```python
from build123d import *

# Parameters (mm, degrees)
SKETCH_1_W      = 90
SKETCH_1_H      = 36
SKETCH_1_R      = 6
EXTRUDE_1_DEPTH = 16
EXTRUDE_2_DEPTH = 20
FILLET_1_R      = 1
FILLET_2_R      = 1


with BuildPart() as part:
    # Эскиз1 → Бобышка-Вытянуть1 (new body)
    with BuildSketch(Plane(origin=(0, 0, 0), x_dir=(1, 0, 0), z_dir=(0, 1, 0))):
        Rectangle(SKETCH_1_W, SKETCH_1_H)
        with Locations(Location((-6, 0, 0), (0, 0, 270))):
            Circle(SKETCH_1_R, mode=Mode.SUBTRACT)
    extrude(amount=EXTRUDE_1_DEPTH)

    # Эскиз3 → Бобышка-Вытянуть2 (add)
    with BuildSketch(Plane(origin=(0, 18, 0), x_dir=(1, 0, 0), z_dir=(0, 1, 0))):
        with BuildLine():
            Line((-45, 20.5), (-45, -20.5))
            Line((-45, -20.5), (-48, -20.5))
            Line((-48, -20.5), (-48, -9.285164832))
            ThreePointArc((-48, -9.285164832), (-48.252071986, -6.546804135), (-48.999815907, -3.900478642))
            Line((-48.999815907, -3.900478642), (-52.000184093, 3.900478642))
            ThreePointArc((-52.000184093, 3.900478642), (-52.747928014, 6.546804135), (-53, 9.285164832))
            Line((-53, 9.285164832), (-53, 19))
            ThreePointArc((-53, 19), (-52.560660172, 20.060660172), (-51.5, 20.5))
            Line((-51.5, 20.5), (-45, 20.5))
        make_face()
    extrude(amount=-EXTRUDE_2_DEPTH)

    # Скругление1
    fillet_1_edges = [part.edges().sort_by_distance(p)[0] for p in [
        (-48.25, 18, -20.5),
        (-52.560660172, 18, -20.060660172),
        (-53, 18, -14.142582416),
        (-52.747928014, 18, -6.546804135),
        (-50.5, 18, 0),
        (-48.252071986, 18, 6.546804135),
        (-48, 18, 14.892582416),
        (-46.5, 18, 20.5),
    ]]
    fillet(fillet_1_edges, radius=FILLET_1_R)

    # Скругление2
    fillet_2_edges = [part.edges().sort_by_distance(p)[0] for p in [
        (-45, -2, 0),
        (-48.25, -2, -20.5),
        (-46.5, -2, 20.5),
        (-48, -2, 14.892582416),
        (-48.252071986, -2, 6.546804135),
        (-50.5, -2, 0),
        (-52.747928014, -2, -6.546804135),
        (-53, -2, -14.142582416),
        (-52.560660172, -2, -20.060660172),
    ]]
    fillet(fillet_2_edges, radius=FILLET_2_R)


solid = part.part
```
Source: CAD feature listing. Evaluate the final solid. Frame: model axes, mm. A direction names the side the tool comes from. Coordinates: 2 decimals unless noted, no trailing zeros. Write each loop counter-clockwise with the first axis right and the second up, starting at its lowest first coordinate (ties: lowest second). Pieces come first, ordered by that corner, then holes. Notation, with made-up numbers: (63, 44.5) - (77, 44.5) arc R34 ccw to (77, 75.5) - close; hole circle Ø5 at (33.25, 44). An arc over 180 degrees is marked (long way). Answer as a JSON object with one key per item and string values.
Q1. Draft query along Z for faces 5 (the cylindrical face through (-11.323, 7.888, 2.769)), 6 (the cylindrical face through (-50.255, -1.699, -0.157)), 7 (the flat face through (-48, -2, -5)). Return one class per face: released by +Z, released by -Z, zero draft, split by the parting line, or undercut.
Ans:
{"face 5": "undercut", "face 6": "released by +Z", "face 7": "zero draft"}
Q2. Section query B-B, the plane y = 14. Output: boundary loops of the cut face in (x, z), plus the area to 3 significant figures.
Ans:
{"outline": "(-53, -19) arc R1.5 ccw to (-51.5, -20.5) - (-45, -20.5) - (-45, -18) - (45, -18) - (45, 18) - (-45, 18) - (-45, 20.5) - (-48, 20.5) - (-48, 9.29) arc R15 cw to (-49, 3.9) - (-52, -3.9) arc R15 ccw to (-53, -9.29) - close; hole circle Ø12 at (-6, 0)", "area": "3,350 mm2"}
Q3. Material intervals for line 1 (Z direction, x = 15, y = 12); line 2 (Y direction, x = -1, z = -3.5); line 3 (X direction, y = 5.25, z = 0), sorted ascending. Write a range as [from, to].
Ans:
{"line 1": "z = [-18, 18]", "line 2": "y = [0, 16]", "line 3": "x = [-50.5, -12], [0, 45]"}
Q4. First-contact query: pin 1 Ø1 at (x, y) = (-17.5, 12.5) entering from +Z; pin 2 Ø2 at (y, z) = (7, 7.5) entering from -X; pin 3 Ø1.5 at (x, y) = (-39.5, 10) entering from -Z. Flat tips, straight axial feed; report the tip coordinate or a pass-through.
Ans:
{"pin 1": "stops at z = 18", "pin 2": "stops at x = -48.26", "pin 3": "stops at z = -18"}
Q5. Section query A-A, the plane x = -6. Output: boundary loops of the cut face in (y, z), plus the area to 3 significant figures.
Ans:
{"outline": "(0, -18) - (16, -18) - (16, -6) - (0, -6) - close; (0, 6) - (16, 6) - (16, 18) - (0, 18) - close", "area": "384 mm2"}
Q6. Set-up query: faces 1 (the flat face through (-1, 8, -18)), 2 (the flat face through (-48, 8, 15)), 3 (the flat face through (-1, 16, -4)), 4 (the flat face through (-1, 0, -4)). Return all of +Z, -Z, +X, -X, +Y, -Y with unobstructed straight access to the full face (end or side cutting, diameter ignored); none if empty.
Ans:
{"face 1": "-Z, +X, +Y, -Y", "face 2": "+Z, -X, +Y, -Y", "face 3": "+Z, -Z, +X, +Y", "face 4": "+Z, -Z, +X, -Y"}
Q7. Section query C-C, the plane z = -13.5. Output: boundary loops of the cut face in (x, y).
Ans:
{"outline": "(-53, -1) arc R1 ccw to (-52, -2) - (-46, -2) arc R1 ccw to (-45, -1) - (-45, 0) - (45, 0) - (45, 16) - (-45, 16) - (-45, 18) - (-52, 18) arc R1 ccw to (-53, 17) - close"}
Q8. Section query D-D, the plane x = 28. Output: boundary loops of the cut face in (y, z), plus the area to 3 significant figures.
Ans:
{"outline": "(0, -18) - (16, -18) - (16, 18) - (0, 18) - close", "area": "576 mm2"}
